Autodesk Inventor part; units mm, degrees
ref_plane "WorkPlane1" through (0, 0, 0) normal (0, 0, 1) x (1, 0, 0)
ref_plane "MSC_PF1" through (0, 0, 0) normal (1, 0, 0) x (0, 1, 0)
ref_plane "MSC_PT1" through (0, 0, 0) normal (0, 0, -1) x (-1, 0, 0)
ref_plane "WorkPlane1" through (0, 0, 0) normal (0, 0, 1) x (1, 0, 0)
sketch "Sketch1" plane through (0, 0, 0) normal (0, 0, 1) x (1, 0, 0)
  point P0 (0, 0)
sketch "Sketch2" plane through (0, 0, 0) normal (0, 0, 1) x (1, 0, 0)
  line L0 (-6.5, 3.7529) -> (-6.5, -3.7529)
  line L1 (0, 7.5054) -> (-6.5, 3.7529)
  line L2 (6.5, 3.7529) -> (0, 7.5054)
  line L3 (6.5, -3.7529) -> (6.5, 3.7529)
  line L4 (0, -7.5054) -> (6.5, -3.7529)
  line L5 (-6.5, -3.7529) -> (0, -7.5054)
  circle A0 centre (0, 0) radius 6.5 construction
  dimension "d1" = 13
  dimension "d29" = 0
  dimension "d30" = 0
extrude "Extrusion1" add sketch "Sketch2" along normal blind 5.3
sketch "Sketch3" plane through (0, 0, 0) normal (1, 0, 0) x (0, 1, 0)
  line L0 (6.5, 5.3) -> (7.6054, 5.3)
  line L1 (7.6054, 4.6618) -> (6.5, 5.3)
  line L2 (7.6054, 5.3) -> (7.6054, 4.6618)
  line L3 (0, -1.06) -> (0, 6.36)
  line L4 (7.5054, 0) -> (7.5054, 5.3)
  dimension "d25" = 0.1
  dimension "d26" = 0
  dimension "d27" = 60
  dimension "d28" = 6.5
revolve "Revolution1" cut sketch "Sketch3" angle 360 about axis through (0, 0, -10) along (0, 0, 1)
sketch "Sketch4" plane through (0, 0, 0) normal (1, 0, 0) x (0, 1, 0)
  line L0 (0, -40) -> (0, 0)
  line L1 (-4, -40) -> (0, -40)
  line L2 (-4, 0) -> (-4, -40)
  line L3 (0, 0) -> (-4, 0)
  line L4 (0, -40) -> (0, 0)
  line L5 (-4.8, 0) -> (0.8, 0)
  line L6 (0, -48) -> (0, 8)
  dimension "d18" = 4
  dimension "d20" = 40
  dimension "d33" = 0
  dimension "d34" = 0
revolve "Revolution2" add sketch "Sketch4" angle 360 about axis through (0, 0, -40) along (0, 0, -1)
chamfer "Chamfer1" distance 0.625 angle 45 1 edges at (0, 4, -40)
fillet "Fillet1" radius 0.4 1 edges at (0, 4, 0)
thread "Thread1"
ref_plane "MSC_PF1" through (0, 0, 0) normal (1, 0, 0) x (0, 1, 0)
ref_plane "MSC_PT1" through (0, 0, 0) normal (0, 0, -1) x (-1, 0, 0)
equation "\"d22\" = 0.5 * PTC"
equation "\"d23\" = 0.5 * PTC"
equation "\"d24\" = r"
equation "\"d1\" = ParS"
equation "\"d6\" = ParK"
equation "\"b\" = NLG - 2 * PTC"
equation "\"d28\" = 0.5 * ParS"
equation "\"d18\" = 0.5 * NND"
equation "\"d20\" = NLG"
equation "\"NND\" = 8"
equation "\"NLG\" = 40"
equation "\"PTC\" = 1.25"
equation "\"ParK\" = 5.3"
equation "\"ParS\" = 13"
equation "\"msp_es\" = 0.577367 * ParS"
equation "\"r\" = 0.4"
equation "\"THREADDIA\" = NND"
properties part number "ISO 4018 - M8 x 40(1)" material "Steel"
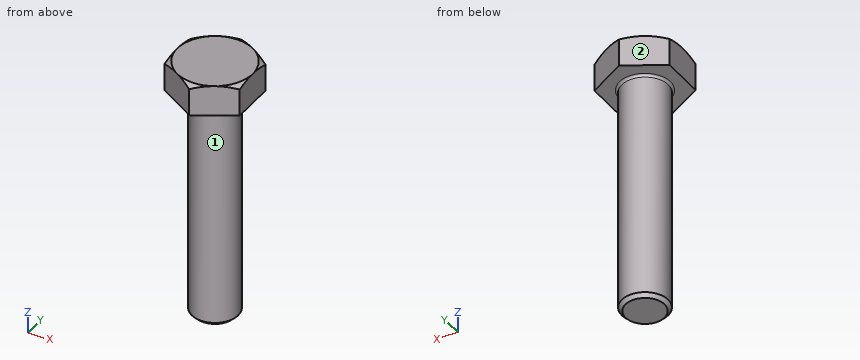
Here's how the part is built. I have some questions about the finished solid (model axes, mm). Face numbers are marked on the shaded views. A direction names the side the tool comes from. Coordinates: 2 decimals unless noted, no trailing zeros. Write each loop counter-clockwise with the first axis right and the second up, starting at its lowest first coordinate (ties: lowest second). Pieces come first, ordered by that corner, then holes. Notation, with made-up numbers: M 17.25,56 L 70.25,56 A15 cw 70.25,63 Z; hole C 24.5,88.25 d5. An arc over 180 degrees is marked long. Answer as CSV lines item,"result". Start each with the question number.
Q1. I need wall thicknesses on probe 1 along Z at (x, y) = (5.5, 1); probe 2 along Y at (x, z) = (0.25, -14.5); probe 3 along Y at (x, z) = (-3.5, 2.5). Which ranges of each line are inside material? Lowest first, please. Write a range as [from, to].
Q2. For the marked faces 1 and 2, which set-ups out of +Z, -Z, +X, -X, +Y, -Y let a thin tool reach every point of the face, with its end or its side?
Q3. Suppose I cut it at A-A, the plane z = 1.5. List the corners of the cut face in (x, y) for me.
Q4. Suppose I cut it at B-B, the plane z = -9. List the corners of the cut face in (x, y) for me, then the cut area to 3 significant figures.
Q5. Will these pins go through, and if not, where does the flat tip stop? pin 1 Ø5 at (y, z) = (1.5, -15) entering from +X; pin 2 Ø8 at (y, z) = (-5.5, -4.5) entering from -X; pin 3 Ø2 at (y, z) = (6, -33.5) entering from -X; pin 4 Ø3 at (y, z) = (-5.5, -1) entering from -X.
Entries:
1,probe 1,"z = [0, 5.3]"
1,probe 2,"y = [-3.99, 3.99]"
1,probe 3,"y = [-5.48, 5.48]"
2,face 1,"-Z"
2,face 2,"+Z, -Z, -X, +Y"
3,outline,"M -6.5,-3.75 L 0,-7.51 L 6.5,-3.75 L 6.5,3.75 L 0,7.51 L -6.5,3.75 Z"
4,outline,"C 0,0 d8"
4,area,"50.3 mm²"
5,pin 1,"stops at x = 4"
5,pin 2,"stops at x = -3.71"
5,pin 3,"passes through"
5,pin 4,"stops at x = -5.41"
